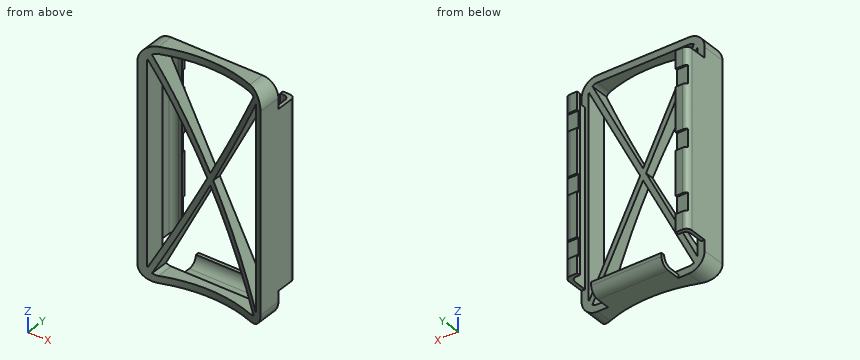
```python
from build123d import *

# Parameters (mm, degrees)
F1_DEPTH      = 25
F2_R          = 75
F3_DEPTH      = 65.001
F3_DEPTH_BACK = 65.001
F5_DEPTH      = 50
F7_DEPTH      = 20
F8_W          = 1
F8_H          = 10
F9_DEPTH      = 35.0010001
F9_DEPTH_BACK = 35.0010001


with BuildPart() as f1:
    # F0 (on Front) → F1 (new body)
    with BuildSketch(Plane.XZ):
        with BuildLine():
            Line((26, 65), (-26, 65))
            ThreePointArc((-26, 65), (-32.3639610307, 62.3639610307), (-35, 56))
            Line((-35, 56), (-35, -56))
            ThreePointArc((-35, -56), (-32.3639610307, -62.3639610307), (-26, -65))
            Line((-26, -65), (26, -65))
            ThreePointArc((26, -65), (32.3639610307, -62.3639610307), (35, -56))
            Line((35, -56), (35, 56))
            ThreePointArc((35, 56), (32.3639610307, 62.3639610307), (26, 65))
        make_face()
        with BuildLine():
            ThreePointArc((-28.8605034902, 60.1009169441), (-27.4992356852, 60.7699363057), (-26, 61))
            Line((-26, 61), (26, 61))
            ThreePointArc((26, 61), (27.4992356852, 60.7699363057), (28.8605034902, 60.1009169441))
            Line((28.8605034902, 60.1009169441), (29.6627722225, 61.6795747722))
            ThreePointArc((29.6627722225, 61.6795747722), (31.6795747722, 62.3372277775), (32.3372277775, 60.3204252278))
            Line((32.3372277775, 60.3204252278), (30.8190334092, 57.333010503))
            ThreePointArc((30.8190334092, 57.333010503), (30.9545517984, 56.6726191174), (31, 56))
            Line((31, 56), (31, -56))
            ThreePointArc((31, -56), (30.9545517984, -56.6726191174), (30.8190334092, -57.333010503))
            Line((30.8190334092, -57.333010503), (32.3372277775, -60.3204252278))
            ThreePointArc((32.3372277775, -60.3204252278), (31.6795747722, -62.3372277775), (29.6627722225, -61.6795747722))
            Line((29.6627722225, -61.6795747722), (28.8605034902, -60.1009169441))
            ThreePointArc((28.8605034902, -60.1009169441), (27.4992356852, -60.7699363057), (26, -61))
            Line((26, -61), (-26, -61))
            ThreePointArc((-26, -61), (-27.4992356852, -60.7699363057), (-28.8605034902, -60.1009169441))
            Line((-28.8605034902, -60.1009169441), (-29.6627722225, -61.6795747722))
            ThreePointArc((-29.6627722225, -61.6795747722), (-31.6795747722, -62.3372277775), (-32.3372277775, -60.3204252278))
            Line((-32.3372277775, -60.3204252278), (-30.8190334092, -57.333010503))
            ThreePointArc((-30.8190334092, -57.333010503), (-30.9545517984, -56.6726191174), (-31, -56))
            Line((-31, -56), (-31, 56))
            ThreePointArc((-31, 56), (-30.9545517984, 56.6726191174), (-30.8190334092, 57.333010503))
            Line((-30.8190334092, 57.333010503), (-32.3372277775, 60.3204252278))
            ThreePointArc((-32.3372277775, 60.3204252278), (-31.6795747722, 62.3372277775), (-29.6627722225, 61.6795747722))
            Line((-29.6627722225, 61.6795747722), (-28.8605034902, 60.1009169441))
        make_face(mode=Mode.SUBTRACT)
        with BuildLine():
            Line((-0.8412927243, -1.6554469737), (-1.6825854486, 0))
            Line((-1.6825854486, 0), (-30.8190334092, -57.333010503))
            ThreePointArc((-30.8190334092, -57.333010503), (-30.4840056321, -58.2121694083), (-29.9902146421, -59.0130030054))
            Line((-29.9902146421, -59.0130030054), (-0.8412927243, -1.6554469737))
        make_face()
        with BuildLine():
            Line((-0.8412927243, 1.6554469737), (-29.9902146421, 59.0130030054))
            ThreePointArc((-29.9902146421, 59.0130030054), (-30.4840056321, 58.2121694083), (-30.8190334092, 57.333010503))
            Line((-30.8190334092, 57.333010503), (-1.6825854486, 0))
            Line((-1.6825854486, 0), (-0.8412927243, 1.6554469737))
        make_face()
        with BuildLine():
            ThreePointArc((30.8190334092, 57.333010503), (30.4840056321, 58.2121694083), (29.9902146421, 59.0130030054))
            Line((29.9902146421, 59.0130030054), (0.8412927243, 1.6554469737))
            Line((0.8412927243, 1.6554469737), (1.6825854486, 0))
            Line((1.6825854486, 0), (30.8190334092, 57.333010503))
        make_face()
        with BuildLine():
            Line((30.8190334092, -57.333010503), (1.6825854486, 0))
            Line((1.6825854486, 0), (0.8412927243, -1.6554469737))
            Line((0.8412927243, -1.6554469737), (29.9902146421, -59.0130030054))
            ThreePointArc((29.9902146421, -59.0130030054), (30.4840056321, -58.2121694083), (30.8190334092, -57.333010503))
        make_face()
        with BuildLine():
            Line((0, -3.3108939473), (-0.8412927243, -1.6554469737))
            Line((-0.8412927243, -1.6554469737), (-29.9902146421, -59.0130030054))
            ThreePointArc((-29.9902146421, -59.0130030054), (-29.4682811184, -59.6015310749), (-28.8605034902, -60.1009169441))
            Line((-28.8605034902, -60.1009169441), (0, -3.3108939473))
        make_face()
        with BuildLine():
            Line((0, 3.3108939473), (-28.8605034902, 60.1009169441))
            ThreePointArc((-28.8605034902, 60.1009169441), (-29.4682811184, 59.6015310749), (-29.9902146421, 59.0130030054))
            Line((-29.9902146421, 59.0130030054), (-0.8412927243, 1.6554469737))
            Line((-0.8412927243, 1.6554469737), (0, 3.3108939473))
        make_face()
        with BuildLine():
            ThreePointArc((29.9902146421, 59.0130030054), (29.4682811184, 59.6015310749), (28.8605034902, 60.1009169441))
            Line((28.8605034902, 60.1009169441), (0, 3.3108939473))
            Line((0, 3.3108939473), (0.8412927243, 1.6554469737))
            Line((0.8412927243, 1.6554469737), (29.9902146421, 59.0130030054))
        make_face()
        with BuildLine():
            Line((29.9902146421, -59.0130030054), (0.8412927243, -1.6554469737))
            Line((0.8412927243, -1.6554469737), (0, -3.3108939473))
            Line((0, -3.3108939473), (28.8605034902, -60.1009169441))
            ThreePointArc((28.8605034902, -60.1009169441), (29.4682811184, -59.6015310749), (29.9902146421, -59.0130030054))
        make_face()
        with BuildLine():
            ThreePointArc((-29.9902146421, -59.0130030054), (-30.4840056321, -58.2121694083), (-30.8190334092, -57.333010503))
            Line((-30.8190334092, -57.333010503), (-32.3372277775, -60.3204252278))
            ThreePointArc((-32.3372277775, -60.3204252278), (-31.6795747722, -62.3372277775), (-29.6627722225, -61.6795747722))
            Line((-29.6627722225, -61.6795747722), (-28.8605034902, -60.1009169441))
            ThreePointArc((-28.8605034902, -60.1009169441), (-29.4682811184, -59.6015310749), (-29.9902146421, -59.0130030054))
        make_face()
        with BuildLine():
            ThreePointArc((-29.9902146421, 59.0130030054), (-29.4682811184, 59.6015310749), (-28.8605034902, 60.1009169441))
            Line((-28.8605034902, 60.1009169441), (-29.6627722225, 61.6795747722))
            ThreePointArc((-29.6627722225, 61.6795747722), (-31.6795747722, 62.3372277775), (-32.3372277775, 60.3204252278))
            Line((-32.3372277775, 60.3204252278), (-30.8190334092, 57.333010503))
            ThreePointArc((-30.8190334092, 57.333010503), (-30.4840056321, 58.2121694083), (-29.9902146421, 59.0130030054))
        make_face()
        with BuildLine():
            Line((29.6627722225, 61.6795747722), (28.8605034902, 60.1009169441))
            ThreePointArc((28.8605034902, 60.1009169441), (29.4682811184, 59.6015310749), (29.9902146421, 59.0130030054))
            ThreePointArc((29.9902146421, 59.0130030054), (30.4840056321, 58.2121694083), (30.8190334092, 57.333010503))
            Line((30.8190334092, 57.333010503), (32.3372277775, 60.3204252278))
            ThreePointArc((32.3372277775, 60.3204252278), (31.6795747722, 62.3372277775), (29.6627722225, 61.6795747722))
        make_face()
        with BuildLine():
            Line((32.3372277775, -60.3204252278), (30.8190334092, -57.333010503))
            ThreePointArc((30.8190334092, -57.333010503), (30.4840056321, -58.2121694083), (29.9902146421, -59.0130030054))
            ThreePointArc((29.9902146421, -59.0130030054), (29.4682811184, -59.6015310749), (28.8605034902, -60.1009169441))
            Line((28.8605034902, -60.1009169441), (29.6627722225, -61.6795747722))
            ThreePointArc((29.6627722225, -61.6795747722), (31.6795747722, -62.3372277775), (32.3372277775, -60.3204252278))
        make_face()
        Polygon((0.8412927243, 1.6554469737), (0, 3.3108939473), (-0.8412927243, 1.6554469737), (0, 0), align=None)
        Polygon((0, 0), (-0.8412927243, 1.6554469737), (-1.6825854486, 0), (-0.8412927243, -1.6554469737), align=None)
        Polygon((1.6825854486, 0), (0.8412927243, 1.6554469737), (0, 0), (0.8412927243, -1.6554469737), align=None)
        Polygon((0.8412927243, -1.6554469737), (0, 0), (-0.8412927243, -1.6554469737), (0, -3.3108939473), align=None)
    extrude(amount=F1_DEPTH)

    # F2 (on Top) → F3 (cut, two sides)
    with BuildSketch(Plane.XY) as f3_sk:
        with Locations((0, -80)):
            Circle(F2_R)
    extrude(amount=-F3_DEPTH, mode=Mode.SUBTRACT)
    extrude(f3_sk.sketch, amount=F3_DEPTH_BACK, mode=Mode.SUBTRACT)

    # F4 (on Top) → F5 (join, symmetric)
    with BuildSketch(Plane.XY):
        with BuildLine():
            Line((-35, 9.8), (-35, 0))
            Line((-35, 0), (-33, 0))
            Line((-33, 0), (-33, 7.8))
            ThreePointArc((-33, 7.8), (-32.1213203436, 9.9213203436), (-30, 10.8))
            Line((-30, 10.8), (-28, 10.8))
            Line((-28, 10.8), (-28, 12.8))
            Line((-28, 12.8), (-32, 12.8))
            ThreePointArc((-32, 12.8), (-34.1213203436, 11.9213203436), (-35, 9.8))
        make_face()
        with BuildLine():
            Line((32, 12.8), (28, 12.8))
            Line((28, 12.8), (28, 10.8))
            Line((28, 10.8), (30, 10.8))
            ThreePointArc((30, 10.8), (32.1213203436, 9.9213203436), (33, 7.8))
            Line((33, 7.8), (33, 0))
            Line((33, 0), (35, 0))
            Line((35, 0), (35, 9.8))
            ThreePointArc((35, 9.8), (34.1213203436, 11.9213203436), (32, 12.8))
        make_face()
    extrude(amount=F5_DEPTH, both=True)

    # F6 (on Right) → F7 (join, symmetric)
    with BuildSketch(Plane.YZ):
        with BuildLine():
            Line((0, -63), (0, -65))
            Line((0, -65), (7.8, -65))
            ThreePointArc((7.8, -65), (11.3355339059, -63.5355339059), (12.8, -60))
            Line((12.8, -60), (12.8, -58))
            Line((12.8, -58), (10.8, -58))
            ThreePointArc((10.8, -58), (9.3355339059, -61.5355339059), (5.8, -63))
            Line((5.8, -63), (0, -63))
        make_face()
    extrude(amount=F7_DEPTH, both=True)

    # F8 (on Right) → F9 (cut, two sides)
    with BuildSketch(Plane.YZ) as f9_sk:
        with Locations((12.3, 35)):
            Rectangle(F8_W, F8_H)
        with Locations((12.3, -35)):
            Rectangle(F8_W, F8_H)
        Polygon((12.8, 5), (11.8, 5), (11.8, -5), (12.8, -5), (12.8, 0), align=None)
    extrude(amount=-F9_DEPTH, mode=Mode.SUBTRACT)
    extrude(f9_sk.sketch, amount=F9_DEPTH_BACK, mode=Mode.SUBTRACT)


solid = f1.part
```
Geometry check sheet. Reference: the model listing, model coordinates, mm. Give positions to 0.01 mm unless a question says otherwise; leave off trailing zeros. Loops run counter-clockwise (first coordinate to the right, second up) from the corner with the lowest first, then second, coordinate; pieces in that order, holes last. Notation, with made-up numbers: M 85,31 L 134,31 A13 ccw 134,51 Z; hole C 10,59.25 d3. An arc over 180 degrees is marked long. Write item = value, one per line. Start each with the question number.
1. Section check A-A, the plane y = 1.5. Enter the section's corners in (x, z).
2. Go/stop test with flat-tipped pins: P1, Ø3.5, axis at x = 31.5, y = 3.5, coming from the +Z side; P2, Ø0.6, axis at y = 11.5, z = -3, coming from the -X side; P3, Ø1.5, axis at x = -9.5, y = 8, coming from the +Z side. Record where each tip stops, or that it passes through.
3. Section check C-C, the plane z = -48. Enter the section's corners in (x, y).
4. Section check D-D, the plane x = -16.5. Enter the section's corners in (y, z), plus the area to 3 significant figures.
5. Thickness scan on probe 1 along X at (y, z) = (2.75, 13); probe 2 along X at (y, z) = (-3.75, -3); probe 3 along Z at (x, y) = (-25.5, -5.5). Record the ranges inside material, lowest first.
6. Section check B-B, the plane x = 10.5. Enter the section's corners in (y, z), plus the area to 3 significant figures.
Values follow:
q1.outline = M -35,-50 L -33,-50 L -33,50 L -35,50 Z; M -20,-65 L 20,-65 L 20,-63 L -20,-63 Z; M 33,-50 L 35,-50 L 35,50 L 33,50 Z
q2.P1 = 50
q2.P2 = -34.65
q2.P3 = -62.04
q3.outline = M -35,-13.67 A75 cw -31,-11.71 L -31,0 L -33,0 L -33,7.8 A3 cw -30,10.8 L -28,10.8 L -28,12.8 L -32,12.8 A3 ccw -35,9.8 Z; M -26.08,-9.68 A75 cw -22.71,-8.52 L -22.71,0 L -26.08,0 Z; M 22.71,-8.52 A75 cw 26.08,-9.68 L 26.08,0 L 22.71,0 Z; M 28,10.8 L 30,10.8 A3 cw 33,7.8 L 33,0 L 31,0 L 31,-11.71 A75 cw 35,-13.67 L 35,9.8 A3 ccw 32,12.8 L 28,12.8 Z
q4.outline = M -6.84,-65 L 7.8,-65 A5 ccw 12.8,-60 L 12.8,-58 L 10.8,-58 A5 cw 5.8,-63 L 0,-63 L 0,-61 L -6.84,-61 Z; M -6.84,-35.78 L 0,-35.78 L 0,-29.16 L -6.84,-29.16 Z; M -6.84,29.16 L 0,29.16 L 0,35.78 L -6.84,35.78 Z; M -6.84,61 L 0,61 L 0,65 L -6.84,65 Z
q4.area = 181 mm^2
q5.probe_1 = -35 to -33, 33 to 35
q5.probe_2 = -35 to -31, -3.21 to 3.21, 31 to 35
q5.probe_3 = -65 to -61, -53.49 to -46.87, 46.87 to 53.49, 61 to 65
q6.outline = M -5.74,-65 L 7.8,-65 A5 ccw 12.8,-60 L 12.8,-58 L 10.8,-58 A5 cw 5.8,-63 L 0,-63 L 0,-61 L -5.74,-61 Z; M -5.74,-23.97 L 0,-23.97 L 0,-17.35 L -5.74,-17.35 Z; M -5.74,17.35 L 0,17.35 L 0,23.97 L -5.74,23.97 Z; M -5.74,61 L 0,61 L 0,65 L -5.74,65 Z
q6.area = 158 mm^2
